Check sheet for the modelled part. Datum: model origin and axes. Units: mm. Give positions to 0.01 mm unless a question says otherwise; leave off trailing zeros. Loops run counter-clockwise (first coordinate to the right, second up) from the corner with the lowest first, then second, coordinate; pieces in that order, holes last. Notation, with made-up numbers: (10, -12.75) -> (55, -12.75) arc R14 cw to (55, 0.25) -> close; hole circle Ø1 at (62.5, 89.25). An arc over 180 degrees is marked (long way). Write each question's results on one line, items separated by ' | '. Start each with the question number.
1. Material ranges on L1, parallel to Z at x = 4.5, y = -5; L2, parallel to X at y = -5.75, z = 1.25; L3, parallel to X at y = 4.5, z = 1, recorded low to high. Write a range as from..to.
2. Gauge pin test, flat ends, axial feed: pin 1 Ø6 at (y, z) = (1, 10) entering from -X; pin 2 Ø2 at (x, z) = (0, 9) entering from +Y; pin 3 Ø1.5 at (x, z) = (-2, 7.5) entering from -Y; pin 4 Ø4 at (y, z) = (0, 10.5) entering from +X. Record the tip position at first contact, or that the pin passes through.
3. Cross-section at B-B on x = -3. Record the boundary of the cut face in (y, z).
4. Cross-section at C-C on y = -6.5. Record the boundary of the cut face in (x, z), and give its area (3 significant figures).
5. Cross-section at A-A on z = 14. Record the boundary of the cut face in (x, y).
from build123d import *

# Parameters (mm, degrees)
SKETCH1_R           = 7.5
BOSS_EXTRUDE1_DEPTH = 2
SKETCH2_R           = 0.25
BOSS_EXTRUDE2_DEPTH = 15
CHAMFER1_SIZE       = 0.25


with BuildPart() as part:
    # Sketch1 → Boss-Extrude1 (new body)
    with BuildSketch(Plane.XY):
        Circle(SKETCH1_R)
    extrude(amount=BOSS_EXTRUDE1_DEPTH)

    # Sketch2 → Boss-Extrude2 (add)
    with BuildSketch(Plane.XY.offset(2)):
        Circle(SKETCH2_R)
    extrude(amount=BOSS_EXTRUDE2_DEPTH)

    # Chamfer1
    chamfer1_edges = [part.edges().sort_by_distance(p)[0] for p in [
        (-0.25, 0, 17),
    ]]
    chamfer(chamfer1_edges, length=CHAMFER1_SIZE)


solid = part.part
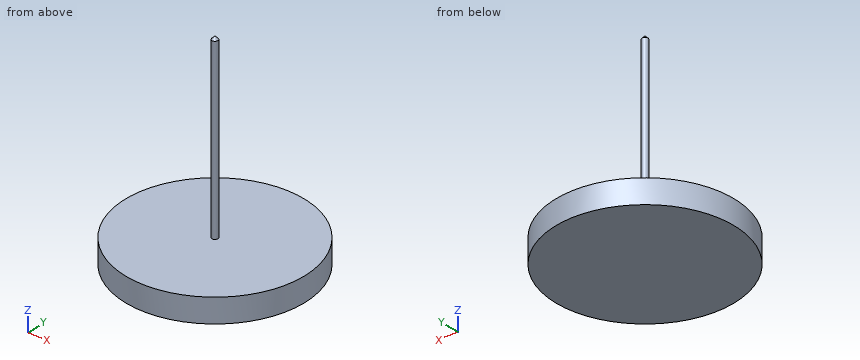
Geometry says:
1) L1: 0..2 | L2: -4.82..4.82 | L3: -6..6
2) pin 1: x = -0.25 | pin 2: y = 0.25 | pin 3: through | pin 4: x = 0.25
3) outline: (-6.87, 0) -> (6.87, 0) -> (6.87, 2) -> (-6.87, 2) -> close
4) outline: (-3.74, 0) -> (3.74, 0) -> (3.74, 2) -> (-3.74, 2) -> close | area: 15.0 mm^2
5) outline: circle Ø0.5 at (0, 0)
